Work out the finished part from the listing and answer in its coordinate system (mm). A direction names the side the tool comes from. Coordinates: 2 decimals unless noted, no trailing zeros. Order: outer loops, then holes, each group sorted by start corner. A loop starts at its lowest first (then second) coordinate and runs counter-clockwise, first axis right, second up. Notation, with made-up numbers: (-0.75, -26.5) -> (58.25, -26.5) arc R11 cw to (58.25, -5.5) -> close; hole circle Ø10 at (52.5, -20). An arc over 180 degrees is marked (long way). Write item = value, one per line. Start each with the question number.
Q1. Straight lines are drawn through the part: L1, parallel to X at y = 43, z = 9; L2, parallel to X at y = 14, z = 9.25; L3, parallel to Y at x = 6.5, z = 2.25. For each, find the intervals that lie inside material, in ascending order. Write a range as from..to.
Q2. The part is cut by section A-A, the plane z = 6. Count the separate pieces of the cut face and the enclosed holes in it, plus the area to 3 significant figures.
Q3. Flat-ended cylindrical pins translate along their axes: pin 1 (6 mm diameter, centred on x = 1.5, y = 75, fed in from -Z) (3 decimals); pin 2 (2 mm diameter, centred on y = 52, z = 5.5, fed in from +X); pin 3 (1.8 mm diameter, centred on x = 5, z = 6, fed in from -Y) (3 decimals); pin 4 (3 mm diameter, centred on y = 29.5, z = 8, fed in from +X). Find the tip coordinate at first contact, or state that the pin passes through.
Q4. Which of the six approach directions +Z, -Z, +X, -X, +Y, -Y give full straight-line access (tool end or side, diameter ignored) to faces 1 (the flat face through (-18.087, 30.018, 6.056)), 2 (the cylindrical face through (6.5, 1.01, 6.07)), 3 (the flat face through (0, 0, 5))?
Q5. The part is cut by section C-C, the plane x = 5. Determine the outline of the cut face in (y, z).
Q6. For a pull along Y with two mould halves and no side action, classify faces 4 (the cylindrical face through (-7.66, 61.84, 6.06)), 5 (the cylindrical face through (19.24, 1.01, 6.07)), 6 (the flat face through (20.014, 40.347, 4.93)) as +Y half, -Y half, draft (parallel to the pull), parting line (faces both ways), or undercut.
Q7. The part is cut by section D-D, the plane y = 22. Determine the outline of the cut face in (x, z), plus the area to 3 significant figures.
Q8. The part is cut by section B-B, the plane x = 0. Determine the outline of the cut face in (y, z), plus the area to 3 significant figures.
```python
from build123d import *

# Parameters (mm, degrees)
SKETCH_1_R          = 10.5
EXTRUDE_1_DEPTH     = 10
CUT_EXTRUDE_2_DEPTH = 8
SKETCH_3_R          = 1.5
CUT_EXTRUDE_3_DEPTH = 97.81941954


with BuildPart() as part:
    # 草图1 → 凸台-拉伸1 (new body)
    with BuildSketch(Plane.XY):
        with BuildLine():
            Line((-25, 0), (25, 0))
            Line((25, 0), (14.88676655, 81.839614547))
            ThreePointArc((14.88676655, 81.839614547), (0, 95), (-14.88676655, 81.839614547))
            Line((-14.88676655, 81.839614547), (-25, 0))
        make_face()
        with Locations((0, 80)):
            Circle(SKETCH_1_R, mode=Mode.SUBTRACT)
    extrude(amount=EXTRUDE_1_DEPTH)

    # 草图2 → 切除-拉伸2 (cut)
    with BuildSketch(Plane.XY.offset(10)):
        with BuildLine():
            Line((-13.564970556, 57.262621959), (-22.737639737, 2))
            Line((-22.737639737, 2), (-1, 2))
            Line((-1, 2), (-2.641694958, 56.527552532))
            ThreePointArc((-2.641694958, 56.527552532), (-7.769922801, 61.84962447), (-13.564970556, 57.262621959))
        make_face()
        with BuildLine():
            Line((2.641694958, 56.527552532), (1, 2))
            Line((1, 2), (22.737639737, 2))
            Line((22.737639737, 2), (13.564970556, 57.262621959))
            ThreePointArc((13.564970556, 57.262621959), (7.769922801, 61.84962447), (2.641694958, 56.527552532))
        make_face()
    extrude(amount=-CUT_EXTRUDE_2_DEPTH, mode=Mode.SUBTRACT)

    # 草图3 → 切除-拉伸3 (cut, through all)
    with BuildSketch(Plane(origin=(0, 2, 0), x_dir=(1, 0, 0), z_dir=(0, 1, 0))):
        with Locations(Location((-17.74, -6, 0), (0, 0, 180))):
            Circle(SKETCH_3_R)
        with Locations(Location((-5, -6, 0), (0, 0, 180))):
            Circle(SKETCH_3_R)
        with Locations(Location((5, -6, 0), (0, 0, 180))):
            Circle(SKETCH_3_R)
        with Locations(Location((17.74, -6, 0), (0, 0, 180))):
            Circle(SKETCH_3_R)
    extrude(amount=-CUT_EXTRUDE_3_DEPTH, mode=Mode.SUBTRACT)


solid = part.part
```
Model answer:
q1.L1 = -19.69..-15.93, -2.23..2.23, 15.93..19.69
q1.L2 = -23.27..-20.75, -1.36..1.36, 20.75..23.27
q1.L3 = 0..2, 61.61..71.75, 88.25..93.52
q2.separate_pieces = 3
q2.enclosed_holes = 1
q2.area = 1,310 mm2
q3.pin_1 = through
q3.pin_2 = 18.7
q3.pin_3 = 60.095
q3.pin_4 = 21.54
q4.face_1 = +Z
q4.face_2 = -Y
q4.face_3 = +Z, -Z, +X, -X, -Y
q5.outline = (0, 0) -> (70.77, 0) -> (70.77, 10) -> (60.88, 10) -> (60.88, 2) -> (2, 2) -> (2, 4.5) -> (0, 4.5) -> close; (0, 7.5) -> (2, 7.5) -> (2, 10) -> (0, 10) -> close; (89.23, 0) -> (94.14, 0) -> (94.14, 10) -> (89.23, 10) -> close
q6.face_4 = undercut
q6.face_5 = draft
q6.face_6 = +Y half
q7.outline = (-22.28, 0) -> (22.28, 0) -> (22.28, 10) -> (19.42, 10) -> (19.42, 2) -> (1.6, 2) -> (1.6, 10) -> (-1.6, 10) -> (-1.6, 2) -> (-19.42, 2) -> (-19.42, 10) -> (-22.28, 10) -> close
q7.area = 161 mm2
q8.outline = (0, 0) -> (69.5, 0) -> (69.5, 10) -> (0, 10) -> close; (90.5, 0) -> (95, 0) -> (95, 10) -> (90.5, 10) -> close
q8.area = 740 mm2
